from build123d import *

# Parameters (mm, degrees)
F1_DEPTH  = 15
F2_R      = 25.5
F3_DEPTH  = 13
F4_DEPTH  = 5
F6_DEPTH  = 25
F8_DEPTH  = 25
F10_DEPTH = 25
F12_DEPTH = 25
F14_DEPTH = 25
F16_DEPTH = 25
F18_DEPTH = 25
F20_DEPTH = 25


with BuildPart() as f1:
    # F0 (on Top) → F1 (new body)
    with BuildSketch(Plane.XY):
        with BuildLine():
            ThreePointArc((27.4715762198, -1.25), (27.4928931366, -0.6251615614), (27.5, 0))
            ThreePointArc((27.5, 0), (27.4928931366, 0.6251615614), (27.4715762198, 1.25))
            ThreePointArc((27.4715762198, 1.25), (25.4066871441, 10.52379439), (20.3092213114, 18.5414543584))
            ThreePointArc((20.3092213114, 18.5414543584), (19.4454364826, 19.4454364826), (18.5414543584, 20.3092213114))
            ThreePointArc((18.5414543584, 20.3092213114), (10.52379439, 25.4066871441), (1.25, 27.4715762198))
            ThreePointArc((1.25, 27.4715762198), (0, 27.5), (-1.25, 27.4715762198))
            ThreePointArc((-1.25, 27.4715762198), (-10.52379439, 25.4066871441), (-18.5414543584, 20.3092213114))
            ThreePointArc((-18.5414543584, 20.3092213114), (-19.4454364826, 19.4454364826), (-20.3092213114, 18.5414543584))
            ThreePointArc((-20.3092213114, 18.5414543584), (-25.4066871441, 10.52379439), (-27.4715762198, 1.25))
            ThreePointArc((-27.4715762198, 1.25), (-27.5, 0), (-27.4715762198, -1.25))
            ThreePointArc((-27.4715762198, -1.25), (-25.4066871441, -10.52379439), (-20.3092213114, -18.5414543584))
            ThreePointArc((-20.3092213114, -18.5414543584), (-19.4454364826, -19.4454364826), (-18.5414543584, -20.3092213114))
            ThreePointArc((-18.5414543584, -20.3092213114), (-10.52379439, -25.4066871441), (-1.25, -27.4715762198))
            ThreePointArc((-1.25, -27.4715762198), (0, -27.5), (1.25, -27.4715762198))
            ThreePointArc((1.25, -27.4715762198), (10.52379439, -25.4066871441), (18.5414543584, -20.3092213114))
            ThreePointArc((18.5414543584, -20.3092213114), (19.4454364826, -19.4454364826), (20.3092213114, -18.5414543584))
            ThreePointArc((20.3092213114, -18.5414543584), (25.4066871441, -10.52379439), (27.4715762198, -1.25))
        make_face()
    extrude(amount=F1_DEPTH)

    # F2 (on face) → F3 (cut)
    with BuildSketch(Plane.XY.offset(15)):
        Circle(F2_R)
    extrude(amount=-F3_DEPTH, mode=Mode.SUBTRACT)

    # F0 (on Top) → F4 (join)
    with BuildSketch(Plane.XY):
        with BuildLine():
            ThreePointArc((-1.25, 27.4715762198), (0, 27.5), (1.25, 27.4715762198))
            Line((1.25, 27.4715762198), (1.25, 39.9715762198))
            Line((1.25, 39.9715762198), (-1.25, 39.9715762198))
            Line((-1.25, 39.9715762198), (-1.25, 27.4715762198))
        make_face()
        with BuildLine():
            ThreePointArc((-20.3092213114, 18.5414543584), (-19.4454364826, 19.4454364826), (-18.5414543584, 20.3092213114))
            Line((-18.5414543584, 20.3092213114), (-27.3802891232, 29.1480560762))
            Line((-27.3802891232, 29.1480560762), (-29.1480560762, 27.3802891232))
            Line((-29.1480560762, 27.3802891232), (-20.3092213114, 18.5414543584))
        make_face()
        with BuildLine():
            ThreePointArc((-27.4715762198, -1.25), (-27.5, 0), (-27.4715762198, 1.25))
            Line((-27.4715762198, 1.25), (-39.9715762198, 1.25))
            Line((-39.9715762198, 1.25), (-39.9715762198, -1.25))
            Line((-39.9715762198, -1.25), (-27.4715762198, -1.25))
        make_face()
        with BuildLine():
            Line((-27.3802891232, -29.1480560762), (-18.5414543584, -20.3092213114))
            ThreePointArc((-18.5414543584, -20.3092213114), (-19.4454364826, -19.4454364826), (-20.3092213114, -18.5414543584))
            Line((-20.3092213114, -18.5414543584), (-29.1480560762, -27.3802891232))
            Line((-29.1480560762, -27.3802891232), (-27.3802891232, -29.1480560762))
        make_face()
        with BuildLine():
            Line((1.25, -39.9715762198), (1.25, -27.4715762198))
            ThreePointArc((1.25, -27.4715762198), (0, -27.5), (-1.25, -27.4715762198))
            Line((-1.25, -27.4715762198), (-1.25, -39.9715762198))
            Line((-1.25, -39.9715762198), (1.25, -39.9715762198))
        make_face()
        with BuildLine():
            Line((29.1480560762, -27.3802891232), (20.3092213114, -18.5414543584))
            ThreePointArc((20.3092213114, -18.5414543584), (19.4454364826, -19.4454364826), (18.5414543584, -20.3092213114))
            Line((18.5414543584, -20.3092213114), (27.3802891232, -29.1480560762))
            Line((27.3802891232, -29.1480560762), (29.1480560762, -27.3802891232))
        make_face()
        with BuildLine():
            ThreePointArc((27.4715762198, 1.25), (27.4928931366, 0.6251615614), (27.5, 0))
            ThreePointArc((27.5, 0), (27.4928931366, -0.6251615614), (27.4715762198, -1.25))
            Line((27.4715762198, -1.25), (39.9715762198, -1.25))
            Line((39.9715762198, -1.25), (39.9715762198, 1.25))
            Line((39.9715762198, 1.25), (27.4715762198, 1.25))
        make_face()
        with BuildLine():
            ThreePointArc((18.5414543584, 20.3092213114), (19.4454364826, 19.4454364826), (20.3092213114, 18.5414543584))
            Line((20.3092213114, 18.5414543584), (29.1480560762, 27.3802891232))
            Line((29.1480560762, 27.3802891232), (27.3802891232, 29.1480560762))
            Line((27.3802891232, 29.1480560762), (18.5414543584, 20.3092213114))
        make_face()
    extrude(amount=F4_DEPTH)

    # F5 (on face) → F6 (cut)
    with BuildSketch(Plane.YZ.offset(1.25)):
        with BuildLine():
            ThreePointArc((-33.4715762198, 2.5), (-34.9715762198, 4), (-36.4715762198, 2.5))
            ThreePointArc((-36.4715762198, 2.5), (-34.9715762198, 1), (-33.4715762198, 2.5))
        make_face()
    extrude(amount=-F6_DEPTH, mode=Mode.SUBTRACT)

    # F7 (on face) → F8 (cut)
    with BuildSketch(Plane(origin=(0.8838834765, -0.8838834765, 0), x_dir=(0.7071067812, 0.7071067812, 0), z_dir=(0.7071067812, -0.7071067812, 0))):
        with BuildLine():
            ThreePointArc((-33.4715762198, 2.5), (-34.9715762198, 4), (-36.4715762198, 2.5))
            ThreePointArc((-36.4715762198, 2.5), (-34.9715762198, 1), (-33.4715762198, 2.5))
        make_face()
    extrude(amount=-F8_DEPTH, mode=Mode.SUBTRACT)

    # F9 (on face) → F10 (cut)
    with BuildSketch(Plane.XZ.offset(1.25)):
        with BuildLine():
            ThreePointArc((-33.4715762198, 2.5), (-34.9715762198, 4), (-36.4715762198, 2.5))
            ThreePointArc((-36.4715762198, 2.5), (-34.9715762198, 1), (-33.4715762198, 2.5))
        make_face()
    extrude(amount=-F10_DEPTH, mode=Mode.SUBTRACT)

    # F11 (on face) → F12 (cut)
    with BuildSketch(Plane(origin=(-0.8838834765, -0.8838834765, 0), x_dir=(0.7071067812, -0.7071067812, 0), z_dir=(-0.7071067812, -0.7071067812, 0))):
        with BuildLine():
            ThreePointArc((-33.4715762198, 2.5), (-34.9715762198, 4), (-36.4715762198, 2.5))
            ThreePointArc((-36.4715762198, 2.5), (-34.9715762198, 1), (-33.4715762198, 2.5))
        make_face()
    extrude(amount=-F12_DEPTH, mode=Mode.SUBTRACT)

    # F13 (on face) → F14 (cut)
    with BuildSketch(Plane(origin=(-1.25, 0, 0), x_dir=(0, -1, 0), z_dir=(-1, 0, 0))):
        with BuildLine():
            ThreePointArc((-33.4715762198, 2.5), (-34.9715762198, 4), (-36.4715762198, 2.5))
            ThreePointArc((-36.4715762198, 2.5), (-34.9715762198, 1), (-33.4715762198, 2.5))
        make_face()
    extrude(amount=-F14_DEPTH, mode=Mode.SUBTRACT)

    # F15 (on face) → F16 (cut)
    with BuildSketch(Plane(origin=(-0.8838834765, 0.8838834765, 0), x_dir=(-0.7071067812, -0.7071067812, 0), z_dir=(-0.7071067812, 0.7071067812, 0))):
        with BuildLine():
            ThreePointArc((-33.4715762198, 2.5), (-34.9715762198, 4), (-36.4715762198, 2.5))
            ThreePointArc((-36.4715762198, 2.5), (-34.9715762198, 1), (-33.4715762198, 2.5))
        make_face()
    extrude(amount=-F16_DEPTH, mode=Mode.SUBTRACT)

    # F17 (on face) → F18 (cut)
    with BuildSketch(Plane(origin=(0, 1.25, 0), x_dir=(-1, 0, 0), z_dir=(0, 1, 0))):
        with BuildLine():
            ThreePointArc((-33.4715762198, 2.5), (-34.9715762198, 4), (-36.4715762198, 2.5))
            ThreePointArc((-36.4715762198, 2.5), (-34.9715762198, 1), (-33.4715762198, 2.5))
        make_face()
    extrude(amount=-F18_DEPTH, mode=Mode.SUBTRACT)

    # F19 (on face) → F20 (cut)
    with BuildSketch(Plane(origin=(0.8838834765, 0.8838834765, 0), x_dir=(-0.7071067812, 0.7071067812, 0), z_dir=(0.7071067812, 0.7071067812, 0))):
        with BuildLine():
            ThreePointArc((-33.4715762198, 2.5), (-34.9715762198, 4), (-36.4715762198, 2.5))
            ThreePointArc((-36.4715762198, 2.5), (-34.9715762198, 1), (-33.4715762198, 2.5))
        make_face()
    extrude(amount=-F20_DEPTH, mode=Mode.SUBTRACT)


solid = f1.part
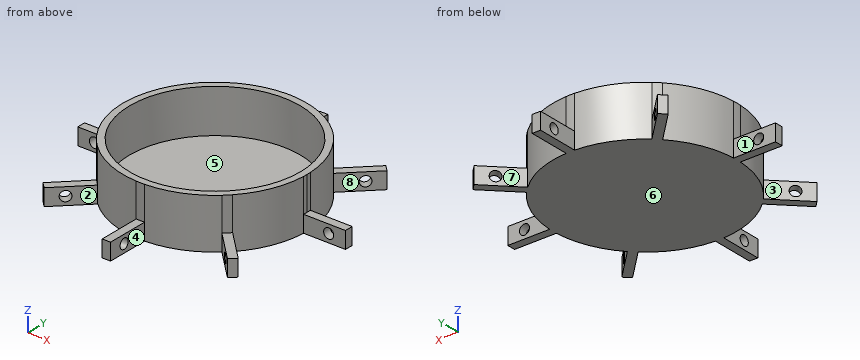
The model under review builds one solid part; all positions refer to its coordinate system, in mm. Face numbers are marked on the shaded views. A direction names the side the tool comes from. Round coordinates to 2 decimals unless told otherwise and drop trailing zeros. Write each loop counter-clockwise with the first axis right and the second up, starting at its lowest first coordinate (ties: lowest second). Pieces come first, ordered by that corner, then holes. Notation, with made-up numbers: M 24,49.25 L 41,49.25 A21 ccw 41,88.25 Z; hole C 8,-38.75 d2. An arc over 180 degrees is marked long. Answer as CSV lines item,"result". Start each with the question number.
Q1. Consider section C-C, the plane x = 14. Give the boundary of the cut face in (y, z).
Q2. Wall thickness on line 1 along Y through (x, z) = (-0.55, 2.5); line 2 along X through (y, z) = (0.1, 2.5); line 3 along Y through (x, z) = (0, 9.5): over which ranges is each line inside the solid? List them lowest first.
Q3. Consider section B-B, the plane y = 12. Give the boundary of the cut face in (x, z), then the cut area to 3 significant figures.
Q4. Tool access review of the marked faces 4, 5, 6, 7 and 8: name each direction out of +Z, -Z, +X, -X, +Y, -Y from which nothing blocks a thin tool from reaching the whole face with its end or side.
Q5. Clearance check with flat-ended pins moving along their axes: P1, Ø2.5, axis at x = 36.5, z = 2.5, coming from the +Y side; P2, Ø5, axis at y = -19.5, z = 9.5, coming from the -X side; P3, Ø2.5, axis at y = -33, z = 2.5, coming from the +X side; P4, Ø3, axis at x = 21.5, y = 26.5, coming from the +Z side. State where each tip first meets the part, or that it passes through.
Q6. Consider section A-A, the plane x = 0. Give the boundary of the cut face in (y, z).
Q7. The part is to be moulded in two halves that separate along X. For the marked faces 1, 2 and 3, say which applies: +X half, -X half, draft (parallel to the pull), parting line (faces both ways), or undercut.
Result set:
1,outline,"M -23.67,0 L 23.67,0 L 23.67,15 L 21.31,15 L 21.31,2 L -21.31,2 L -21.31,15 L -23.67,15 Z"
2,line 1,"y = -39.97 to -36.47, -33.47 to -25.49, 25.49 to 33.47, 36.47 to 39.97"
2,line 2,"x = -39.97 to -36.47, -33.47 to -25.5, 25.5 to 33.47, 36.47 to 39.97"
2,line 3,"y = -27.5 to -25.5, 25.5 to 27.5"
3,outline,"M -24.74,0 L 24.74,0 L 24.74,15 L 22.5,15 L 22.5,2 L -22.5,2 L -22.5,15 L -24.74,15 Z"
3,area,"157 mm²"
4,face 4,"+Z, -Z, -Y"
4,face 5,"+Z"
4,face 6,"-Z, +X, -X, +Y, -Y"
4,face 7,"+Z, -Z, +Y"
4,face 8,"+Z, -Z, +X"
5,P1,"stops at y = 1.25"
5,P2,"stops at x = -21.62"
5,P3,"stops at x = 1.25"
5,P4,"passes through"
6,outline,"M -39.97,0 L 39.97,0 L 39.97,5 L 27.5,5 L 27.5,15 L 25.5,15 L 25.5,2 L -25.5,2 L -25.5,15 L -27.5,15 L -27.5,5 L -39.97,5 Z; hole C -34.97,2.5 d3; hole C 34.97,2.5 d3"
7,face 1,"draft"
7,face 2,"undercut"
7,face 3,"-X half"
